from build123d import *

# Parameters (mm, degrees)
SKETCH_1_W          = 96
SKETCH_1_H          = 60
EXTRUDE_1_DEPTH     = 10
FILLET_1_R          = 10
SKETCH_2_R          = 2.12
CUT_EXTRUDE_1_DEPTH = 10
SKETCH_3_R          = 5
CUT_EXTRUDE_2_DEPTH = 5
SKETCH_4_R          = 3.1
CUT_EXTRUDE_3_DEPTH = 5
CHAMFER_1_SIZE      = 1
CHAMFER_2_SIZE      = 1
SKETCH_5_W          = 50
SKETCH_5_H          = 20
CUT_EXTRUDE_4_DEPTH = 10
FILLET_2_R          = 10
CHAMFER_3_SIZE      = 2


with BuildPart() as part:
    # 草图1 → 凸台-拉伸1 (new body)
    with BuildSketch(Plane.XY):
        Rectangle(SKETCH_1_W, SKETCH_1_H)
    extrude(amount=EXTRUDE_1_DEPTH)

    # 圆角1
    fillet_1_edges = [part.edges().sort_by_distance(p)[0] for p in [
        (48, -30, 5),
        (-48, -30, 5),
        (-48, 30, 5),
        (48, 30, 5),
    ]]
    fillet(fillet_1_edges, radius=FILLET_1_R)

    # 草图2 → 切除-拉伸1 (cut)
    with BuildSketch(Plane.XY.offset(10)):
        with Locations((0, 17.3)):
            Circle(SKETCH_2_R)
        with Locations((-12.7, 17.3)):
            Circle(SKETCH_2_R)
        with Locations(Location((12.7, 17.3, 0), (0, 0, 180))):
            Circle(SKETCH_2_R)
        with Locations((-12.7, -20.8)):
            Circle(SKETCH_2_R)
        with Locations((0, -20.8)):
            Circle(SKETCH_2_R)
        with Locations((12.7, -20.8)):
            Circle(SKETCH_2_R)
    extrude(amount=-CUT_EXTRUDE_1_DEPTH, mode=Mode.SUBTRACT)

    # 草图3 → 切除-拉伸2 (cut)
    with BuildSketch(Plane.XY.offset(10)):
        with Locations((-38, 20)):
            Circle(SKETCH_3_R)
        with Locations((-38, 0)):
            Circle(SKETCH_3_R)
        with Locations((-38, -20)):
            Circle(SKETCH_3_R)
        with Locations(Location((38, -20, 0), (0, 0, 180))):
            Circle(SKETCH_3_R)
        with Locations(Location((38, 0, 0), (0, 0, 180))):
            Circle(SKETCH_3_R)
        with Locations(Location((38, 20, 0), (0, 0, 180))):
            Circle(SKETCH_3_R)
    extrude(amount=-CUT_EXTRUDE_2_DEPTH, mode=Mode.SUBTRACT)

    # 草图4 → 切除-拉伸3 (cut)
    with BuildSketch(Plane.XY.offset(5)):
        with Locations((-38, 20)):
            Circle(SKETCH_4_R)
        with Locations((-38, 0)):
            Circle(SKETCH_4_R)
        with Locations((-38, -20)):
            Circle(SKETCH_4_R)
        with Locations((38, 20)):
            Circle(SKETCH_4_R)
        with Locations((38, 0)):
            Circle(SKETCH_4_R)
        with Locations((38, -20)):
            Circle(SKETCH_4_R)
    extrude(amount=-CUT_EXTRUDE_3_DEPTH, mode=Mode.SUBTRACT)

    # 倒角1
    chamfer_1_edges = [part.edges().sort_by_distance(p)[0] for p in [
        (-41.1, 0, 0),
        (-41.1, -20, 0),
        (34.9, 20, 0),
        (34.9, 0, 0),
        (34.9, -20, 0),
        (-41.1, 20, 0),
    ]]
    chamfer(chamfer_1_edges, length=CHAMFER_1_SIZE)

    # 倒角2
    chamfer_2_edges = [part.edges().sort_by_distance(p)[0] for p in [
        (0, 30, 10),
        (48, 0, 10),
        (-48, 0, 10),
        (0, -30, 10),
        (-45.071067812, -27.071067812, 10),
        (45.071067812, -27.071067812, 10),
        (-45.071067812, 27.071067812, 10),
        (45.071067812, 27.071067812, 10),
    ]]
    chamfer(chamfer_2_edges, length=CHAMFER_2_SIZE)

    # 草图5 → 切除-拉伸4 (cut)
    with BuildSketch(Plane.XY.offset(10)):
        Rectangle(SKETCH_5_W, SKETCH_5_H)
    extrude(amount=-CUT_EXTRUDE_4_DEPTH, mode=Mode.SUBTRACT)

    # 圆角2
    fillet_2_edges = [part.edges().sort_by_distance(p)[0] for p in [
        (25, -10, 5),
        (25, 10, 5),
        (-25, -10, 5),
        (-25, 10, 5),
    ]]
    fillet(fillet_2_edges, radius=FILLET_2_R - 0.0001)  # a hair under: the kernel refuses the full size

    # 倒角3
    chamfer_3_edges = [part.edges().sort_by_distance(p)[0] for p in [
        (0, -10, 10),
        (0, -10, 0),
        (0, 10, 10),
        (0, 10, 0),
        (22.071097101, -7.071097101, 10),
        (22.071097101, -7.071097101, 0),
        (22.071097101, 7.071097101, 10),
        (22.071097101, 7.071097101, 0),
        (-22.071097101, -7.071097101, 10),
        (-22.071097101, -7.071097101, 0),
        (-22.071097101, 7.071097101, 10),
        (-22.071097101, 7.071097101, 0),
    ]]
    chamfer(chamfer_3_edges, length=CHAMFER_3_SIZE)


solid = part.part
Here's how the part is built. I have some questions about the finished solid (model axes, mm). A direction names the side the tool comes from. Round coordinates to 2 decimals unless told otherwise and drop trailing zeros. Loops run counter-clockwise (first coordinate to the right, second up) from the corner with the lowest first, then second, coordinate; pieces in that order, holes last.
1. If we section it at B-B on x = 12.7: Write out the boundary of the cut face in (y, z).
Answer list:
outline: (-30, 0) - (-22.92, 0) - (-22.92, 10) - (-29, 10) - (-30, 9) - close; (-18.68, 0) - (-12, 0) - (-10, 2) - (-10, 8) - (-12, 10) - (-18.68, 10) - close; (10, 2) - (12, 0) - (15.18, 0) - (15.18, 10) - (12, 10) - (10, 8) - close; (19.42, 0) - (30, 0) - (30, 9) - (29, 10) - (19.42, 10) - close
2. We'd pull the mould along X, two halves only. Please class faces 1 (the face through (-44.548, 26.405, 9.84)), 2 (the face through (-35.136, -21.187, 3.028)), 3 (the face through (-1, -30, 4)), 4 (the face through (42, -17, 8)): +X half, -X half, draft (parallel to the pull), parting line (faces both ways), or undercut.
Answer list:
face 1: -X half
face 2: undercut
face 3: draft
face 4: undercut
3. Which directions (+Z, -Z, +X, -X, +Y, -Y) give clear straight access to the entire face, cutting with the end or side of a thin tool? Please do faces 5 (the face through (-22.372, 7.536, 1.458)), 6 (the face through (44.99, -27.15, 4.56)), 7 (the face through (43, 0, 8)), 8 (the face through (0, -10, 5)).
Answer list:
face 5: -Z
face 6: +Z, -Z, +X, -Y
face 7: +Z
face 8: +Z, -Z
4. If we section it at A-A on x = -8: Write out the boundary of the cut face in (y, z), plus the area to 3 significant figures.
Answer list:
outline: (-30, 0) - (-12, 0) - (-10, 2) - (-10, 8) - (-12, 10) - (-29, 10) - (-30, 9) - close; (10, 2) - (12, 0) - (30, 0) - (30, 9) - (29, 10) - (12, 10) - (10, 8) - close
area: 391 mm2
5. For P1, Ø3.5, axis at x = 12.7, y = 17.3, coming from the +Z side; P2, Ø7, axis at x = 38, y = 0, coming from the -Z side; P3, Ø8, axis at x = 38, y = 20, coming from the +Z side, each with a flat end and sliding along its axis, tell me the tip position at first contact or that it passes through.
Answer list:
P1: passes through
P2: stops at z = 0.6
P3: stops at z = 5
6. If I drill on line 1 along Y through (x, z) = (38, 8.85); line 2 along Y through (x, z) = (38, 3.7); line 3 along X through (y, z) = (19, 3.25), over which ranges is the centre line in solid material (lowest first)?
Answer list:
line 1: y = -30 to -25, -15 to -5, 5 to 15, 25 to 30
line 2: y = -30 to -23.1, -16.9 to -3.1, 3.1 to 16.9, 23.1 to 30
line 3: x = -48 to -40.93, -35.07 to -13.97, -11.43 to -1.27, 1.27 to 11.43, 13.97 to 35.07, 40.93 to 48
